```python
from build123d import *

# Parameters (mm, degrees)
ESQUISSE1_W      = 105
ESQUISSE1_H      = 100
ESQUISSE1_R      = 1.5
EXTRUSION1_DEPTH = 3
ESQUISSE2_W      = 45
ESQUISSE2_H      = 45
EXTRUSION2_DEPTH = 15
CONG_1_R         = 2
ESQUISSE3_W      = 5
ESQUISSE3_H      = 10
ESQUISSE3_W_2    = 10
ESQUISSE3_H_2    = 5
EXTRUSION3_DEPTH = 15
ESQUISSE4_W      = 25
ESQUISSE4_H      = 10
EXTRUSION4_DEPTH = 20


with BuildPart() as part:
    # Esquisse1 → Extrusion1 (new body)
    with BuildSketch(Plane(origin=(0, 0, 0), x_dir=(1, 0, 0), z_dir=(0, 1, 0))):
        with Locations((52.5, 50)):
            Rectangle(ESQUISSE1_W, ESQUISSE1_H)
        with Locations((5, 95)):
            Circle(ESQUISSE1_R, mode=Mode.SUBTRACT)
        with Locations((100, 95)):
            Circle(ESQUISSE1_R, mode=Mode.SUBTRACT)
        with Locations((100, 5)):
            Circle(ESQUISSE1_R, mode=Mode.SUBTRACT)
        with Locations((5, 5)):
            Circle(ESQUISSE1_R, mode=Mode.SUBTRACT)
    extrude(amount=EXTRUSION1_DEPTH)

    # Esquisse2 → Extrusion2 (add)
    with BuildSketch(Plane(origin=(0, 3, 0), x_dir=(1, 0, 0), z_dir=(0, 1, 0))):
        with Locations((36.405733266, 27.475906062)):
            Rectangle(ESQUISSE2_W, ESQUISSE2_H)
    extrude(amount=EXTRUSION2_DEPTH)

    # Congé1
    cong_1_edges = [part.edges().sort_by_distance(p)[0] for p in [
        (13.905733266, 18, -27.475906062),
        (36.405733266, 18, -4.975906062),
        (58.905733266, 18, -27.475906062),
        (36.405733266, 18, -49.975906062),
    ]]
    fillet(cong_1_edges, radius=CONG_1_R)

    # Esquisse3 → Extrusion3 (add)
    with BuildSketch(Plane(origin=(0, 3, 0), x_dir=(1, 0, 0), z_dir=(0, 1, 0))):
        with Locations((97.027568737, 70.884369428)):
            Rectangle(ESQUISSE3_W, ESQUISSE3_H)
        with Locations((13.884436985, 83.782819762)):
            Rectangle(ESQUISSE3_W_2, ESQUISSE3_H_2)
        with Locations((13.884436985, 73.782819762)):
            Rectangle(ESQUISSE3_W_2, ESQUISSE3_H_2)
        with Locations((13.884436985, 63.782819762)):
            Rectangle(ESQUISSE3_W_2, ESQUISSE3_H_2)
        with Locations((97.027568737, 50.884369428)):
            Rectangle(ESQUISSE3_W, ESQUISSE3_H)
        with Locations((97.027568737, 30.884369428)):
            Rectangle(ESQUISSE3_W, ESQUISSE3_H)
    extrude(amount=EXTRUSION3_DEPTH)

    # Esquisse4 → Extrusion4 (add)
    with BuildSketch(Plane(origin=(0, 3, 0), x_dir=(1, 0, 0), z_dir=(0, 1, 0))):
        with Locations((43.077660713, 85.165216912)):
            Rectangle(ESQUISSE4_W, ESQUISSE4_H)
        with Locations((43.077660713, 70.165216912)):
            Rectangle(ESQUISSE4_W, ESQUISSE4_H)
    extrude(amount=EXTRUSION4_DEPTH)


solid = part.part
```
Geometry check sheet. Reference: the model listing, model coordinates, mm. A direction names the side the tool comes from. Round coordinates to 2 decimals unless told otherwise and drop trailing zeros. Loops run counter-clockwise (first coordinate to the right, second up) from the corner with the lowest first, then second, coordinate; pieces in that order, holes last. Notation, with made-up numbers: (83, -17) - (123, -17) arc R26 cw to (123, -3) - close; hole circle Ø4 at (-25.5, -16). An arc over 180 degrees is marked (long way). Write each question's results on one line, items separated by ' | '. Start each with the question number.
Q1. Thickness scan on line 1 (X direction, y = 0.6, z = -95); line 2 (Z direction, x = 5, y = 2.3); line 3 (Z direction, x = 48, y = 4). Record the ranges inside material, lowest first. Write a range as [from, to].
Q2. Access from +Z, -Z, +X, -X, +Y, -Y to the whole of each face (thin tool, end or side, straight path). Record for faces 1 (the flat face through (99.528, 10, -31)), 2 (the flat face through (94.528, 10, -31)), 3 (the flat face through (8.884, 10, -74)), 4 (the flat face through (14, 10, -71.283)), 5 (the flat face through (18.884, 10, -84)).
Q3. Cross-section at A-A on z = -95. Enter the section's corners in (x, y).
Q4. Cross-section at B-B on x = 5. Enter the section's corners in (y, z).
Q5. Gauge pin test, flat ends, axial feed: P1, Ø10, axis at x = 45, y = 15, coming from the +Z side; P2, Ø2.5, axis at y = 9.5, z = -74.5, coming from the +X side; P3, Ø8, axis at y = 9.5, z = -83.5, coming from the +X side. Record the tip position at first contact, or that the pin passes through.
Q6. Cross-section at D-D on x = 35. Enter the section's corners in (y, z), and give its area (3 significant figures).
Q7. Cross-section at C-C on z = -22.5. Enter the section's corners in (x, y).
Q8. Release check for a two-part mould opening along X. For faces 6 (the flat face through (97, 10, -35.884)), 7 (the flat face through (13.906, 9, -27)), 8 (the flat face through (30.578, 13, -70)), 9 (the flat face through (99.528, 10, -71)) record: +X half, -X half, draft (parallel to the pull), parting line (faces both ways), or undercut.
Answers below:
1) line 1: x = [0, 3.5], [6.5, 98.5], [101.5, 105] | line 2: z = [-100, -96.5], [-93.5, -6.5], [-3.5, 0] | line 3: z = [-90.17, -80.17], [-75.17, -65.17], [-49.98, -4.98]
2) face 1: +Z, -Z, +X, +Y | face 2: +Z, -Z, +Y | face 3: +Z, -Z, -X, +Y | face 4: -X, +Y | face 5: -Z, +Y
3) outline: (0, 0) - (3.5, 0) - (3.5, 3) - (0, 3) - close; (6.5, 0) - (98.5, 0) - (98.5, 3) - (6.5, 3) - close; (101.5, 0) - (105, 0) - (105, 3) - (101.5, 3) - close
4) outline: (0, -100) - (3, -100) - (3, -96.5) - (0, -96.5) - close; (0, -93.5) - (3, -93.5) - (3, -6.5) - (0, -6.5) - close; (0, -3.5) - (3, -3.5) - (3, 0) - (0, 0) - close
5) P1: stops at z = -4.98 | P2: stops at x = 99.53 | P3: stops at x = 55.58
6) outline: (0, -100) - (3, -100) - (3, -90.17) - (23, -90.17) - (23, -80.17) - (3, -80.17) - (3, -75.17) - (23, -75.17) - (23, -65.17) - (3, -65.17) - (3, -49.98) - (16, -49.98) arc R2 ccw to (18, -47.98) - (18, -6.98) arc R2 ccw to (16, -4.98) - (3, -4.98) - (3, 0) - (0, 0) - close | area: 1,370 mm²
7) outline: (0, 0) - (105, 0) - (105, 3) - (58.91, 3) - (58.91, 16) arc R2 ccw to (56.91, 18) - (15.91, 18) arc R2 ccw to (13.91, 16) - (13.91, 3) - (0, 3) - close
8) face 6: draft | face 7: -X half | face 8: undercut | face 9: +X half
